from build123d import *

# Parameters (mm, degrees)
BOSS_EXTRUDE1_DEPTH = 54
SKETCH2_W           = 3
SKETCH2_H           = 9.1
CUT_EXTRUDE1_DEPTH  = 27
SKETCH3_W           = 26
SKETCH3_H           = 25
BOSS_EXTRUDE2_DEPTH = 1.5


with BuildPart() as part:
    # Sketch1 → Boss-Extrude1 (new body)
    with BuildSketch(Plane.XY):
        Polygon((-13, 67), (-13, 0), (13, 0), (13, 67), (10, 67), (10, 51), (9.8, 51), (9.8, 19), (8, 19), (8, 2), (-8, 2), (-8, 19), (-9.8, 19), (-9.8, 51), (-10, 51), (-10, 67), align=None)
    extrude(amount=BOSS_EXTRUDE1_DEPTH)

    # Sketch2 → Cut-Extrude1 (cut, through all)
    with BuildSketch(Plane(origin=(13, 0, 0), x_dir=(0, 0, -1), z_dir=(1, 0, 0))):
        Polygon((-45.6, 57.9), (-45.6, 67), (-54, 67), (-54, 0), (-34.2, 0), (-34.2, 57.9), (-34.2, 67), (-42.6, 67), (-42.6, 57.9), align=None)
        with Locations((-32.7, 62.45)):
            Rectangle(SKETCH2_W, SKETCH2_H)
        with Locations((-21.3, 62.45)):
            Rectangle(SKETCH2_W, SKETCH2_H)
        with Locations((-9.9, 62.45)):
            Rectangle(SKETCH2_W, SKETCH2_H)
        with Locations((-44.1, 62.45)):
            Rectangle(SKETCH2_W, SKETCH2_H)
    extrude(amount=-CUT_EXTRUDE1_DEPTH, mode=Mode.SUBTRACT)

    # Sketch3 → Boss-Extrude2 (add)
    with BuildSketch(Plane(origin=(0, 0, 0), x_dir=(-1, 0, 0), z_dir=(0, 0, -1))):
        with Locations((0, 12.5)):
            Rectangle(SKETCH3_W, SKETCH3_H)
    extrude(amount=BOSS_EXTRUDE2_DEPTH)


solid = part.part
The listing builds one solid part. Answer for the finished solid, in the listing's coordinates (mm). A direction names the side the tool comes from. Round coordinates to 2 decimals unless told otherwise and drop trailing zeros. Loops run counter-clockwise (first coordinate to the right, second up) from the corner with the lowest first, then second, coordinate; pieces in that order, holes last. Notation, with made-up numbers: M 1,65 L 42,65 A23 cw 42,82 Z; hole C -10.5,-28 d2. An arc over 180 degrees is marked long. Write each question's results on one line, items separated by ' | '. Start each with the question number.
1) Which of the six approach directions +Z, -Z, +X, -X, +Y, -Y give full straight-line access (tool end or side, diameter ignored) to faces 1 (the flat face through (12, 57.9, 33)), 2 (the flat face through (12, 57.9, 10)), 3 (the flat face through (-10, 59, 17))?
2) Find section B-B on z = 18. Write down the section's boundary in (x, y).
3) Straight lines are drawn through the part: probe 1 along X at (y, z) = (4, 3.5); probe 2 along X at (y, z) = (55.5, 16); probe 3 along Y at (x, z) = (-8.5, 21.5). For each, find the intervals that lie inside material, in ascending order.
4) Each of these flat-tipped pins is pushed along its axis until it touches: pin 1 (6 mm diameter, centred on x = -1.5, z = 29.5, fed in from -Y); pin 2 (2.5 mm diameter, centred on x = 11.5, y = 61.5, fed in from -Z); pin 3 (12 mm diameter, centred on x = -3, y = 45, fed in from +Z); pin 4 (1.5 mm diameter, centred on x = 11.5, y = 60.5, fed in from +Z). Where does it stop, or does it pass through?
5) Find section A-A on y = 34. Write down the section's boundary in (x, z), plus the area to 3 significant figures.
6) Find section C-C on x = 7.25. Write down the section's boundary in (y, z), plus the area to 3 significant figures.
7) Find section D-D on y = 56.5. Write down the section's boundary in (x, z).
8) Determine the mould class of faces 4 (the flat face through (-11, 67, 4)), 5 (the flat face through (-11, 62, 22.8)), 6 (the flat face through (12, 62, 31.2)) for opening direction Z: pulls with the +Z half, pulls with the -Z half, needs draft (parallel to the pull), parting line crosses it, or undercut.
Final values:
1) face 1: +Z, +X, -X, +Y | face 2: +X, -X, +Y | face 3: +Z, -Z, +Y
2) outline: M -13,0 L 13,0 L 13,67 L 10,67 L 10,51 L 9.8,51 L 9.8,19 L 8,19 L 8,2 L -8,2 L -8,19 L -9.8,19 L -9.8,51 L -10,51 L -10,67 L -13,67 Z
3) probe 1: -13 to -8, 8 to 13 | probe 2: -13 to -10, 10 to 13 | probe 3: 0 to 19
4) pin 1: y = 0 | pin 2: z = 0 | pin 3: through | pin 4: z = 31.2
5) outline: M -13,0 L -9.8,0 L -9.8,34.2 L -13,34.2 Z; M 9.8,0 L 13,0 L 13,34.2 L 9.8,34.2 Z | area: 219 mm²
6) outline: M 0,-1.5 L 25,-1.5 L 25,0 L 2,0 L 2,34.2 L 0,34.2 Z | area: 106 mm²
7) outline: M -13,0 L -10,0 L -10,34.2 L -13,34.2 Z; M 10,0 L 13,0 L 13,34.2 L 10,34.2 Z
8) face 4: needs draft | face 5: undercut | face 6: pulls with the +Z half
